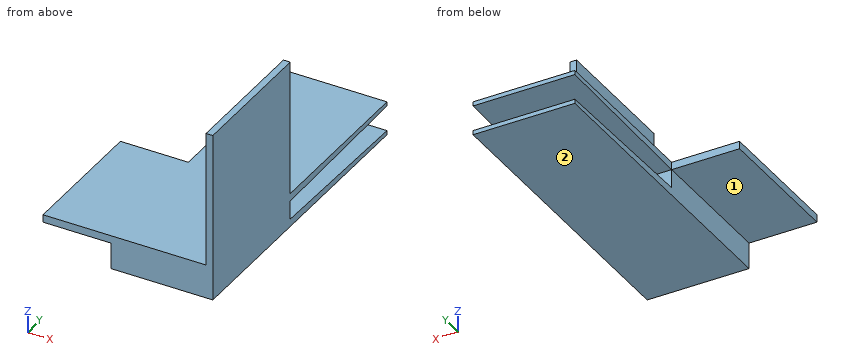
```python
from build123d import *

# Parameters (mm, degrees)
F0_W     = 30
F0_H     = 10
F1_DEPTH = 40
F2_W     = 30
F2_H     = 2.25
F3_DEPTH = 50
F5_DEPTH = 30
F6_W     = 40
F6_H     = 2.25
F7_DEPTH = 20
F8_W     = 2
F8_H     = 40
F9_DEPTH = 40


with BuildPart() as f1:
    # F0 (on Front) → F1 (new body)
    with BuildSketch(Plane.XZ):
        with Locations((15, 5)):
            Rectangle(F0_W, F0_H)
    extrude(amount=F1_DEPTH)

    # F2 (on face) → F3 (join)
    with BuildSketch(Plane(origin=(0, 0, 0), x_dir=(-1, 0, 0), z_dir=(0, 1, 0))):
        with Locations((-15, 8.875)):
            Rectangle(F2_W, F2_H)
        with Locations((-15, 1.125)):
            Rectangle(F2_W, F2_H)
    extrude(amount=F3_DEPTH)

    # F4 (on face) → F5 (cut, through all)
    with BuildSketch(Plane(origin=(0, 0, 0), x_dir=(0, -1, 0), z_dir=(-1, 0, 0))):
        Polygon((-50, 7.75), (0, 7.75), (-50, 8.75), align=None)
        Polygon((-50, 1.25), (0, 2.25), (-50, 2.25), align=None)
    extrude(amount=-F5_DEPTH, mode=Mode.SUBTRACT)

    # F6 (on face) → F7 (join)
    with BuildSketch(Plane(origin=(0, 0, 0), x_dir=(0, -1, 0), z_dir=(-1, 0, 0))):
        with Locations((20, 8.875)):
            Rectangle(F6_W, F6_H)
    extrude(amount=F7_DEPTH)

    # F8 (on face) → F9 (join)
    with BuildSketch(Plane.XY.offset(10)):
        with Locations((29, -20)):
            Rectangle(F8_W, F8_H)
    extrude(amount=F9_DEPTH)


solid = f1.part
```
Build history of the part. All positions in model axes, mm. Face numbers are marked on the shaded views. A direction names the side the tool comes from. Coordinates: 2 decimals unless noted, no trailing zeros. Order: outer loops, then holes, each group sorted by start corner. A loop starts at its lowest first (then second) coordinate and runs counter-clockwise, first axis right, second up.
Item 1: Drill centre lines: L1, parallel to Z at x = 17.5, y = 0.5; L2, parallel to Z at x = 13, y = -31; L3, parallel to Y at x = 9, z = 4. Where is each one in solid material? Low to high.
Filled in:
L1: z = 0 to 2.24, 7.76 to 10
L2: z = 0 to 10
L3: y = -40 to 0
Item 2: Saw through at D-D on y = 2. List the corners of the cut face in (x, z).
Filled in:
outline: (0, 0) - (30, 0) - (30, 2.21) - (0, 2.21) - close; (0, 7.79) - (30, 7.79) - (30, 10) - (0, 10) - close
Item 3: Drop flat-ended pins along their axis: pin 1 Ø1.6 at (x, z) = (15, 4) entering from +Y; pin 2 Ø1.5 at (x, y) = (-14, -16.5) entering from +Z; pin 3 Ø1.8 at (y, z) = (30, 8.5) entering from -X. Give the stop position or say it passes through.
Filled in:
pin 1: stops at y = 0
pin 2: stops at z = 10
pin 3: stops at x = 0
Item 4: Tool access for the marked faces 1 and 2: list every direction of +Z, -Z, +X, -X, +Y, -Y with a clear straight run to the whole face (end or side of a thin tool).
Filled in:
face 1: -Z, -X, +Y, -Y
face 2: -Z, +X, -X, +Y, -Y
Item 5: Saw through at A-A on y = 27.5. List the corners of the cut face in (x, z), then the cut area to 3 significant figures.
Filled in:
outline: (0, 0) - (30, 0) - (30, 1.7) - (0, 1.7) - close; (0, 8.3) - (30, 8.3) - (30, 10) - (0, 10) - close
area: 102 mm2
Item 6: Saw through at B-B on y = -24. List the corners of the cut face in (x, z), then the cut area to 3 significant figures.
Filled in:
outline: (-20, 7.75) - (0, 7.75) - (0, 0) - (30, 0) - (30, 50) - (28, 50) - (28, 10) - (-20, 10) - close
area: 425 mm2
Item 7: Saw through at C-C on x = 24. List the corners of the cut face in (y, z).
Filled in:
outline: (-40, 0) - (50, 0) - (50, 1.25) - (0, 2.25) - (0, 7.75) - (50, 8.75) - (50, 10) - (-40, 10) - close
